Build history of the part. All positions in model axes, mm. A direction names the side the tool comes from. Round coordinates to 2 decimals unless told otherwise and drop trailing zeros. Loops run counter-clockwise (first coordinate to the right, second up) from the corner with the lowest first, then second, coordinate; pieces in that order, holes last. Notation, with made-up numbers: (-6, 19.25) -> (33, 19.25) arc R18 cw to (33, 48.25) -> close; hole circle Ø2 at (30.25, 11.25). An arc over 180 degrees is marked (long way). Put each result on its own line as item: value. Start each with the question number.
Item 1: Cut at A-A, the plane z = 91. List the corners of the cut face in (x, y).
Item 2: Cut at D-D, the plane z = 207. List the corners of the cut face in (x, y).
Item 3: Cut at C-C, the plane x = 0. List the corners of the cut face in (y, z), plus the area to 3 significant figures.
Item 4: Cut at B-B, the plane y = 0. List the corners of the cut face in (x, z).
Item 5: Pull direction Y, two halves, no side cores. Call faces 1 (the flat face through (-5, -325, 168)), 2 (the flat face through (544, 2, 190)), 3 (the flat face through (-350, -2, 419)): +Y half, -Y half, draft (parallel to the pull), parting line (faces both ways), or undercut.
Item 6: Tool access for faces 4 (the flat face through (350, -2, 419)), 5 (the flat face through (-5, -216, 340)), 6 (the flat face through (-539, 2, 190)), 7 (the flat face through (-200, -17, 59)): list every direction of +Z, -Z, +X, -X, +Y, -Y with a clear straight run to the whole face (end or side of a thin tool).
Item 7: Flat gauge pins, fed straight in: pin 1 Ø10 at (x, y) = (468, -216.5) entering from +Z; pin 2 Ø8 at (y, z) = (187.5, 403) entering from +X. Where does each tip first touch, or does it go through?
Item 8: Drill centre lines: probe 1 along X at (y, z) = (-120, 98); probe 2 along Y at (x, z) = (0, 216); probe 3 along Y at (x, z) = (0, 400). Where is each one in solid material? Low to high. Write a range as [from, to].
```python
from build123d import *

# Parameters (mm, degrees)
F0_W      = 1200
F0_H      = 600
F1_DEPTH  = 340
F3_DEPTH  = 150
F5_DEPTH  = 150
F6_W      = 700
F6_H      = 400
F7_DEPTH  = 160
F8_R      = 110
F9_DEPTH  = 500.001
F10_DEPTH = 25
F11_W     = 400
F11_H     = 120
F12_DEPTH = 625.001
F13_R     = 60


with BuildPart() as f1:
    # F0 (on Top) → F1 (new body)
    with BuildSketch(Plane.XY):
        with Locations((3.413781058, 0)):
            Rectangle(F0_W, F0_H)
    extrude(amount=F1_DEPTH)

    # F2 (on face) → F3 (cut)
    with BuildSketch(Plane.XY.offset(340)):
        with BuildLine():
            ThreePointArc((-596.586218942, -150), (-490.520201764, -106.066017178), (-446.586218942, 0))
            ThreePointArc((-446.586218942, 0), (-490.520201764, 106.066017178), (-596.586218942, 150))
            Line((-596.586218942, 150), (-596.586218942, -150))
        make_face()
    extrude(amount=-F3_DEPTH, mode=Mode.SUBTRACT)

    # F4 (on face) → F5 (cut)
    with BuildSketch(Plane.XY.offset(340)):
        with BuildLine():
            Line((603.413781058, -150), (603.413781058, 150))
            ThreePointArc((603.413781058, 150), (453.413781058, 0), (603.413781058, -150))
        make_face()
    extrude(amount=-F5_DEPTH, mode=Mode.SUBTRACT)

    # F6 (on face) → F7 (join)
    with BuildSketch(Plane.XY.offset(340)):
        Rectangle(F6_W, F6_H)
    extrude(amount=F7_DEPTH)

    # F8 (on face) → F9 (cut, through all)
    with BuildSketch(Plane.XY.offset(500)):
        Circle(F8_R)
    extrude(amount=-F9_DEPTH, mode=Mode.SUBTRACT)

    # F10 (add): a face of the model
    f10_faces = [f1.faces().sort_by_distance(p)[0] for p in [
        (3.413781058, -300, 170),
    ]]
    extrude(f10_faces, amount=F10_DEPTH)

    # F11 (on face) → F12 (cut, through all)
    with BuildSketch(Plane.XZ.offset(325)):
        with Locations((0, 60)):
            Rectangle(F11_W, F11_H)
    extrude(amount=-F12_DEPTH, mode=Mode.SUBTRACT)

    # F13
    f13_edges = [f1.edges().sort_by_distance(p)[0] for p in [
        (-350, -200, 420),
        (350, -200, 420),
        (350, 200, 420),
        (-350, 200, 420),
    ]]
    fillet(f13_edges, radius=F13_R)


solid = f1.part
```
Reply:
1. outline: (-596.59, -325) -> (-200, -325) -> (-200, 300) -> (-596.59, 300) -> close; (200, -325) -> (603.41, -325) -> (603.41, 300) -> (200, 300) -> close
2. outline: (-596.59, -325) -> (603.41, -325) -> (603.41, -150) arc R150 cw to (603.41, 150) -> (603.41, 300) -> (-596.59, 300) -> (-596.59, 150) arc R150 cw to (-596.59, -150) -> close; hole circle Ø220 at (0, 0)
3. outline: (-325, 120) -> (-110, 120) -> (-110, 500) -> (-200, 500) -> (-200, 340) -> (-325, 340) -> close; (110, 120) -> (300, 120) -> (300, 340) -> (200, 340) -> (200, 500) -> (110, 500) -> close
3. area: 118,000 mm^2
4. outline: (-596.59, 0) -> (-200, 0) -> (-200, 120) -> (-110, 120) -> (-110, 500) -> (-350, 500) -> (-350, 340) -> (-446.59, 340) -> (-446.59, 190) -> (-596.59, 190) -> close; (110, 120) -> (200, 120) -> (200, 0) -> (603.41, 0) -> (603.41, 190) -> (453.41, 190) -> (453.41, 340) -> (350, 340) -> (350, 500) -> (110, 500) -> close
5. face 1: -Y half
5. face 2: undercut
5. face 3: draft
6. face 4: +Z, +X, +Y, -Y
6. face 5: +Z
6. face 6: +Z, -X
6. face 7: -Z, +Y, -Y
7. pin 1: stops at z = 340
7. pin 2: stops at x = 331.32
8. probe 1: x = [-596.59, -200], [200, 603.41]
8. probe 2: y = [-325, -110], [110, 300]
8. probe 3: y = [-200, -110], [110, 200]
